Check sheet for the modelled part. Datum: model origin and axes. Units: mm. A direction names the side the tool comes from. Round coordinates to 2 decimals unless told otherwise and drop trailing zeros. Order: outer loops, then holes, each group sorted by start corner. A loop starts at its lowest first (then second) coordinate and runs counter-clockwise, first axis right, second up.
Q1. Scan lines: probe 1 along X at (y, z) = (-14, -0.75); probe 2 along Y at (x, z) = (0, 1.25) (3 decimals); probe 3 along Y at (x, z) = (-10.5, 2). Record each from-to range of solid material in increasing order.
Q2. Mould release check, pull along Y, two halves, no side actions. Record for faces 1 (the cylindrical face through (-15.53, -1.46, 0.04)), 2 (the flat face through (0, -4, -3.175)), 3 (the cylindrical face through (-6.05, 16.42, 0.04)): +Y half, -Y half, draft (parallel to the pull), parting line (faces both ways), or undercut.
Q3. Set-up check for faces 4 (the cylindrical face through (4.048, 15.125, 0.044)), 5 (the cylindrical face through (6.62, -14.19, 0.04)), 6 (the cylindrical face through (14.1, 6.69, 0.04)): record each of +Z, -Z, +X, -X, +Y, -Y from which the full face is reachable in a straight line by a thin tool's end or side.
Q4. Cross-section at D-D on z = -2.25. Give the number of separate pieces and of enclosed holes in the cut face, then the cut area to 3 significant figures.
Q5. Cross-section at B-B on y = 15.5. Record the cut outline in (x, z) (3 decimals), then the cut area to 3 significant figures.
Q6. Cross-section at A-A on y = 0. Record the cut outline in (x, z) (1 decimal), then the cut area to 3 significant figures.
Q7. Cross-section at C-C on x = -1. Record the cut outline in (y, z) (3 decimals), then the cut area to 3 significant figures.
Q8. Depth check by flat-ended pin: P1, Ø3, axis at y = -8.5, z = 2, coming from the -X side; P2, Ø3, axis at y = 2, z = -1.5, coming from the -X side. Enter the tip coordinate at first touch or a pass-through.
from build123d import *

# Parameters (mm, degrees)
BOSS_EXTRU_1_DEPTH = 3.175
ESQUISSE2_R        = 3.175
ESQUISSE2_R_2      = 1.83
CUT_EXTRUDE1_DEPTH = 26.426049992


with BuildPart() as part:
    # Esquisse1 → Boss.-Extru.1 (new, symmetric)
    with BuildSketch(Plane.XY):
        with BuildLine():
            ThreePointArc((12.39632517, 5.499582215), (14.117106651, 6.707055833), (15.344833887, 8.413445964))
            ThreePointArc((15.344833887, 8.413445964), (15.119886604, 8.811301214), (14.884626197, 9.203146363))
            ThreePointArc((14.884626197, 9.203146363), (12.79475517, 8.97616501), (10.895903967, 8.074252844))
            ThreePointArc((10.895903967, 8.074252844), (10.353325809, 8.759162457), (9.767767389, 9.407709736))
            ThreePointArc((9.767767389, 9.407709736), (10.97179275, 11.130905713), (11.541859176, 13.154295373))
            ThreePointArc((11.541859176, 13.154295373), (11.194403365, 13.451220514), (10.839311962, 13.73897071))
            ThreePointArc((10.839311962, 13.73897071), (8.953107774, 12.81090002), (7.47724344, 11.313934452))
            ThreePointArc((7.47724344, 11.313934452), (6.733133864, 11.771966302), (5.961072705, 12.18112862))
            ThreePointArc((5.961072705, 12.18112862), (6.503118716, 14.21220409), (6.346765909, 16.308542623))
            ThreePointArc((6.346765909, 16.308542623), (5.918709868, 16.4687241), (5.486616734, 16.617672425))
            ThreePointArc((5.486616734, 16.617672425), (4.031583448, 15.100451419), (3.156717001, 13.18898859))
            ThreePointArc((3.156717001, 13.18898859), (2.300826605, 13.364897275), (1.435384677, 13.485323618))
            ThreePointArc((1.435384677, 13.485323618), (1.25007259, 15.579300904), (0.386159005, 17.495738945))
            ThreePointArc((0.386159005, 17.495738945), (-0.07086739, 17.499856508), (-0.527845446, 17.492037594))
            ThreePointArc((-0.527845446, 17.492037594), (-1.376209343, 15.568665517), (-1.544556096, 13.473256055))
            ThreePointArc((-1.544556096, 13.473256055), (-2.408994299, 13.345824393), (-3.263431928, 13.162989565))
            ThreePointArc((-3.263431928, 13.162989565), (-4.15375074, 15.067304103), (-5.621024374, 16.57269094))
            ThreePointArc((-5.621024374, 16.57269094), (-6.051896994, 16.420247951), (-6.478641676, 16.256604874))
            ThreePointArc((-6.478641676, 16.256604874), (-6.618010975, 14.159068786), (-6.059532932, 12.132449995))
            ThreePointArc((-6.059532932, 12.132449995), (-6.828254938, 11.717048125), (-7.568630479, 11.253004706))
            ThreePointArc((-7.568630479, 11.253004706), (-9.056570428, 12.737968057), (-10.950229256, 13.650731821))
            ThreePointArc((-10.950229256, 13.650731821), (-11.302978505, 13.360115154), (-11.648018105, 13.060385685))
            ThreePointArc((-11.648018105, 13.060385685), (-11.061582813, 11.041679393), (-9.843640668, 9.328291411))
            ThreePointArc((-9.843640668, 9.328291411), (-10.423927257, 8.675022928), (-10.960940493, 7.985741403))
            ThreePointArc((-10.960940493, 7.985741403), (-12.867034061, 8.872245071), (-14.958674882, 9.082292981))
            ThreePointArc((-14.958674882, 9.082292981), (-15.190753994, 8.688555294), (-15.412471643, 8.288891231))
            ThreePointArc((-15.412471643, 8.288891231), (-14.170964512, 6.592500507), (-12.440460063, 5.399003211))
            ThreePointArc((-12.440460063, 5.399003211), (-12.762320108, 4.586661936), (-13.031199317, 3.75527983))
            ThreePointArc((-13.031199317, 3.75527983), (-15.12554349, 3.93639839), (-17.16288355, 3.418395567))
            ThreePointArc((-17.16288355, 3.418395567), (-17.246300359, 2.969027437), (-17.317953638, 2.517634164))
            ThreePointArc((-17.317953638, 2.517634164), (-15.57111875, 1.348168766), (-13.536776372, 0.818515543))
            ThreePointArc((-13.536776372, 0.818515543), (-13.561388802, -0.054918177), (-13.529703184, -0.928123913))
            ThreePointArc((-13.529703184, -0.928123913), (-15.559689144, -1.474236033), (-17.296995165, -2.657810803))
            ThreePointArc((-17.296995165, -2.657810803), (-17.221688373, -3.108608947), (-17.134634839, -3.55728674))
            ThreePointArc((-17.134634839, -3.55728674), (-15.093166261, -4.058772026), (-13.00035767, -3.860697179))
            ThreePointArc((-13.00035767, -3.860697179), (-12.724753862, -4.689874348), (-12.39632517, -5.499582215))
            ThreePointArc((-12.39632517, -5.499582215), (-14.117106651, -6.707055833), (-15.344833887, -8.413445964))
            ThreePointArc((-15.344833887, -8.413445964), (-15.119886604, -8.811301214), (-14.884626197, -9.203146363))
            ThreePointArc((-14.884626197, -9.203146363), (-12.79475517, -8.97616501), (-10.895903967, -8.074252844))
            ThreePointArc((-10.895903967, -8.074252844), (-10.353325809, -8.759162457), (-9.767767389, -9.407709736))
            ThreePointArc((-9.767767389, -9.407709736), (-10.97179275, -11.130905713), (-11.541859176, -13.154295373))
            ThreePointArc((-11.541859176, -13.154295373), (-11.194403365, -13.451220514), (-10.839311962, -13.73897071))
            ThreePointArc((-10.839311962, -13.73897071), (-8.953107774, -12.81090002), (-7.47724344, -11.313934452))
            ThreePointArc((-7.47724344, -11.313934452), (-6.733133864, -11.771966302), (-5.961072705, -12.18112862))
            ThreePointArc((-5.961072705, -12.18112862), (-6.503118716, -14.21220409), (-6.346765909, -16.308542623))
            ThreePointArc((-6.346765909, -16.308542623), (-5.918709868, -16.4687241), (-5.486616734, -16.617672425))
            ThreePointArc((-5.486616734, -16.617672425), (-4.031583448, -15.100451419), (-3.156717001, -13.18898859))
            ThreePointArc((-3.156717001, -13.18898859), (-2.300826605, -13.364897275), (-1.435384677, -13.485323618))
            ThreePointArc((-1.435384677, -13.485323618), (-1.25007259, -15.579300904), (-0.386159005, -17.495738945))
            ThreePointArc((-0.386159005, -17.495738945), (0.07086739, -17.499856508), (0.527845446, -17.492037594))
            ThreePointArc((0.527845446, -17.492037594), (1.376209343, -15.568665517), (1.544556096, -13.473256055))
            ThreePointArc((1.544556096, -13.473256055), (2.408994299, -13.345824393), (3.263431928, -13.162989565))
            ThreePointArc((3.263431928, -13.162989565), (4.15375074, -15.067304103), (5.621024374, -16.57269094))
            ThreePointArc((5.621024374, -16.57269094), (6.051896994, -16.420247951), (6.478641676, -16.256604874))
            ThreePointArc((6.478641676, -16.256604874), (6.618010975, -14.159068786), (6.059532932, -12.132449995))
            ThreePointArc((6.059532932, -12.132449995), (6.828254938, -11.717048125), (7.568630479, -11.253004706))
            ThreePointArc((7.568630479, -11.253004706), (9.056570428, -12.737968057), (10.950229256, -13.650731821))
            ThreePointArc((10.950229256, -13.650731821), (11.302978505, -13.360115154), (11.648018105, -13.060385685))
            ThreePointArc((11.648018105, -13.060385685), (11.061582813, -11.041679393), (9.843640668, -9.328291411))
            ThreePointArc((9.843640668, -9.328291411), (10.423927257, -8.675022928), (10.960940493, -7.985741403))
            ThreePointArc((10.960940493, -7.985741403), (12.867034061, -8.872245071), (14.958674882, -9.082292981))
            ThreePointArc((14.958674882, -9.082292981), (15.190753994, -8.688555294), (15.412471643, -8.288891231))
            ThreePointArc((15.412471643, -8.288891231), (14.170964512, -6.592500507), (12.440460063, -5.399003211))
            ThreePointArc((12.440460063, -5.399003211), (12.762320108, -4.586661936), (13.031199317, -3.75527983))
            ThreePointArc((13.031199317, -3.75527983), (15.12554349, -3.93639839), (17.16288355, -3.418395567))
            ThreePointArc((17.16288355, -3.418395567), (17.246300359, -2.969027437), (17.317953638, -2.517634164))
            ThreePointArc((17.317953638, -2.517634164), (15.57111875, -1.348168766), (13.536776372, -0.818515543))
            ThreePointArc((13.536776372, -0.818515543), (13.561388802, 0.054918177), (13.529703184, 0.928123913))
            ThreePointArc((13.529703184, 0.928123913), (15.559689144, 1.474236033), (17.296995165, 2.657810803))
            ThreePointArc((17.296995165, 2.657810803), (17.221688373, 3.108608947), (17.134634839, 3.55728674))
            ThreePointArc((17.134634839, 3.55728674), (15.093166261, 4.058772026), (13.00035767, 3.860697179))
            ThreePointArc((13.00035767, 3.860697179), (12.724753862, 4.689874348), (12.39632517, 5.499582215))
        make_face()
    extrude(amount=BOSS_EXTRU_1_DEPTH, both=True)

    # Esquisse2 → Cut-Extrude1 (cut, through all)
    with BuildSketch(Plane.XY.offset(3.175)):
        Circle(ESQUISSE2_R)
        with Locations((6.914797213, 6.914797213)):
            Circle(ESQUISSE2_R_2)
        with Locations((6.914797213, -6.914797213)):
            Circle(ESQUISSE2_R_2)
        with Locations((-6.914797213, -6.914797213)):
            Circle(ESQUISSE2_R_2)
        with Locations((-6.914797213, 6.914797213)):
            Circle(ESQUISSE2_R_2)
    extrude(amount=-CUT_EXTRUDE1_DEPTH, mode=Mode.SUBTRACT)


solid = part.part
Results found:
1. probe 1: x = -6.48 to -3.43, -1.46 to 1.57, 3.56 to 6.6
1. probe 2: y = -17.5 to -3.175, 3.175 to 17.5
1. probe 3: y = -13.63 to -10.3, -8.58 to 8.58, 10.1 to 13.5
2. face 1: undercut
2. face 2: draft
2. face 3: +Y half
3. face 4: +Z, -Z, +Y
3. face 5: +Z, -Z
3. face 6: +Z, -Z, +X
4. separate pieces: 1
4. enclosed holes: 5
4. area: 677 mm2
5. outline: (-6.611, -3.175) - (-4.481, -3.175) - (-4.481, 3.175) - (-6.611, 3.175) - close; (-1.393, -3.175) - (1.27, -3.175) - (1.27, 3.175) - (-1.393, 3.175) - close; (4.327, -3.175) - (6.491, -3.175) - (6.491, 3.175) - (4.327, 3.175) - close
5. area: 44.2 mm2
6. outline: (-13.6, -3.2) - (-3.2, -3.2) - (-3.2, 3.2) - (-13.6, 3.2) - close; (3.2, -3.2) - (13.6, -3.2) - (13.6, 3.2) - (3.2, 3.2) - close
6. area: 132 mm2
7. outline: (-16.336, -3.175) - (-3.013, -3.175) - (-3.013, 3.175) - (-16.336, 3.175) - close; (3.013, -3.175) - (16.639, -3.175) - (16.639, 3.175) - (3.013, 3.175) - close
7. area: 171 mm2
8. P1: stops at x = -15.34
8. P2: stops at x = -17.32
